Part print with two shaded views. Sizes in mm from the minimum x, y, z corner. A direction names the side the tool comes from. Give positions to 0.01 mm unless a question says otherwise; leave off trailing zeros. Write each loop counter-clockwise with the first axis right and the second up, starting at its lowest first coordinate (ties: lowest second). Pieces come first, ordered by that corner, then holes. Notation, with made-up numbers: (17, 59.25) -> (75, 59.25) arc R23 ccw to (75, 95.25) -> close; hole circle Ø6 at (26, -15.5). An arc over 180 degrees is marked (long way). Answer as a JSON object with one key per item and string values.
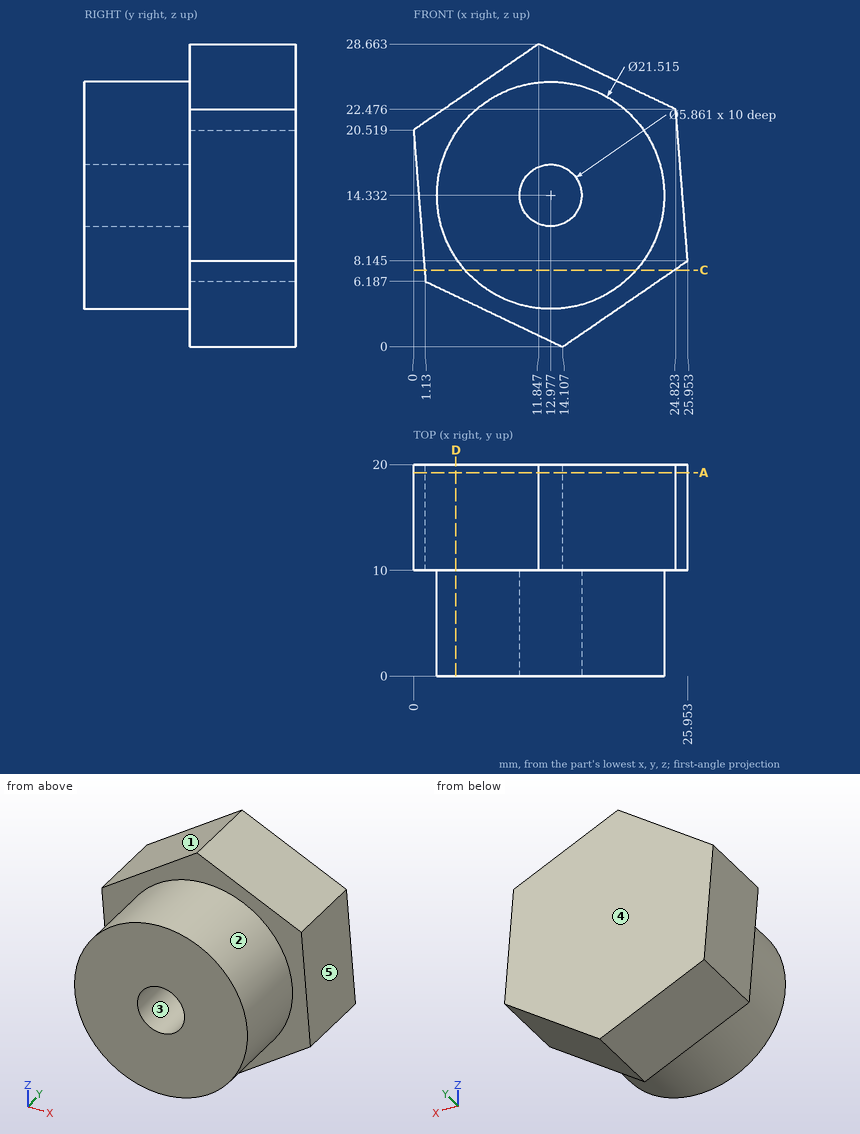
1) Slice it at C-C (z = 7.25). List the corners of the cut face in (x, y) (1 decimal), then the cut area to 3 significant figures.
Model answer:
{"outline": "(1, 10) -> (4.9, 10) -> (4.9, 0) -> (21.1, 0) -> (21.1, 10) -> (24.7, 10) -> (24.7, 20) -> (1, 20) -> close", "area": "398 mm2"}
2) Slice it at A-A (y = 19.25). List the corners of the cut face in (x, z) (1 decimal), then the cut area to 3 significant figures.
Model answer:
{"outline": "(0, 20.5) -> (1.1, 6.2) -> (14.1, 0) -> (26, 8.1) -> (24.8, 22.5) -> (11.8, 28.7) -> close", "area": "537 mm2"}
3) 3-axis set-ups, long thin cutter, end or side, ignore diameter. For the marked faces 1 and 2: which of +Z, -Z, +X, -X, +Y, -Y reach the whole face in a straight line?
Model answer:
{"face 1": "+Z, -X, +Y, -Y", "face 2": "-Y"}
4) Wall check: probe 1 along Z at (x, y) = (13, 5.5) (1 decimal); probe 2 along Y at (x, z) = (4, 21.5); probe 3 along Z at (x, y) = (13.5, 2.5) (1 decimal). Give the ranges that are in metal, low to high.
Model answer:
{"probe 1": "z = 3.6 to 11.4, 17.3 to 25.1", "probe 2": "y = 10 to 20", "probe 3": "z = 3.6 to 11.4, 17.2 to 25.1"}
5) Slice it at D-D (x = 4). List the corners of the cut face in (y, z), then the cut area to 3 significant figures.
Model answer:
{"outline": "(0, 8.4) -> (10, 8.4) -> (10, 4.82) -> (20, 4.82) -> (20, 23.27) -> (10, 23.27) -> (10, 20.26) -> (0, 20.26) -> close", "area": "303 mm2"}
6) Pin check, flat tips, straight feed: pin 1 (3 mm diameter, centred on x = 22.5, y = 4.5, fed in from +Z); pin 2 (6 mm diameter, centred on x = 8, y = 6, fed in from -Z); pin 3 (1 mm diameter, centred on y = 8.5, z = 20, fed in from -X). Stop position of each tip, or through.
Model answer:
{"pin 1": "stops at z = 21.5", "pin 2": "stops at z = 3.76", "pin 3": "stops at x = 3.54"}
7) Mould opens along X. For the marked faces 3, 4 and 5 say: released by +X, released by -X, zero draft, split by the parting line, or undercut.
Model answer:
{"face 3": "undercut", "face 4": "zero draft", "face 5": "released by +X"}
